from build123d import *

# Parameters (mm, degrees)
SKETCH1_R   = 6
SKETCH1_R_2 = 1.25
MAIN_DEPTH  = 8
SKETCH4_R   = 2.5


with BuildPart() as part:
    # Sketch1 → Main (new body)
    with BuildSketch(Plane.XY):
        Circle(SKETCH1_R)
        Circle(SKETCH1_R_2, mode=Mode.SUBTRACT)
    extrude(amount=MAIN_DEPTH)

    # Sketch3 → TopMain (revolve)
    with BuildSketch(Plane(origin=(0, 0, 0), x_dir=(0, 0, -1), z_dir=(1, 0, 0))):
        with BuildLine():
            Line((-8, 0), (-14, 0))
            ThreePointArc((-14, 0), (-12.242640687, -4.242640687), (-8, -6))
            Line((-8, -6), (-8, 0))
        make_face()
    revolve(axis=Axis((0, 0, 10.5), (0, 0, -1)))

    # Sketch4 → HookHole (revolve, cut)
    with BuildSketch(Plane(origin=(0, 0, 0), x_dir=(0, 0, -1), z_dir=(1, 0, 0))):
        with Locations((-7, 0)):
            Circle(SKETCH4_R)
    revolve(axis=Axis((0, 6.6, 13), (0, -1, 0)), mode=Mode.SUBTRACT)


solid = part.part
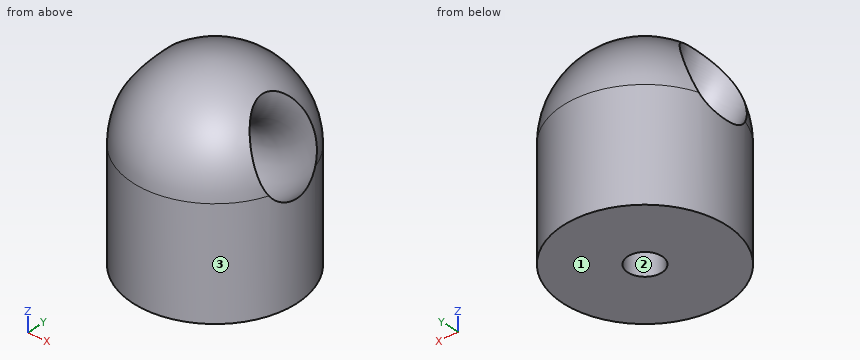
Can you work these out from the model? Positions are in its coordinate system, mm. Face numbers are marked on the shaded views. Coordinates: 2 decimals unless noted, no trailing zeros. Write each loop counter-clockwise with the first axis right and the second up, starting at its lowest first coordinate (ties: lowest second). Pieces come first, ordered by that corner, then holes. Notation, with made-up numbers: (-28.75, 25.5) -> (19.25, 25.5) arc R35 ccw to (19.25, 60.5) -> close; hole circle Ø9 at (74, 20.25). An arc over 180 degrees is marked (long way). Write item = value, one per line.
(1) Imagine slicing it at A-A (y = 0). Please give me the cut outline in (x, z) (3 decimals).
Verdict:
outline = (-6, 0) -> (-1.25, 0) -> (-1.25, 4.592) arc R8.5 cw to (-6, 6.979) -> close; (-3.498, 12.875) arc R3.5 ccw to (3.498, 12.875) arc R6 ccw to start; (1.25, 0) -> (6, 0) -> (6, 6.979) arc R8.5 cw to (1.25, 4.592) -> close
(2) For pin 1 (5 mm diameter, centred on x = -4, y = -3, fed in from +Z); pin 2 (4 mm diameter, centred on y = 2.5, z = 11, fed in from -X); pin 3 (4 mm diameter, centred on y = -2.5, z = 4.5, fed in from -X); pin 4 (6 mm diameter, centred on y = -1, z = 3, fed in from +X), each with a flat end and sliding along its axis, tell me the tip position at first contact or that it passes through.
Verdict:
pin_1 = 13.45
pin_2 = -5.41
pin_3 = -5.98
pin_4 = 6
(3) Imagine slicing it at B-B (z = 3.5). Please give me the cut outline in (x, y), and give its area (3 significant figures).
Verdict:
outline = circle Ø12 at (0, 0); hole circle Ø2.5 at (0, 0)
area = 108 mm^2
(4) Thinking about a two-plate mould opening in X: for the marked faces 1, 2 and 3, which applies, +X half, -X half, draft (parallel to the pull), parting line (faces both ways), or undercut?
Verdict:
face_1 = draft
face_2 = undercut
face_3 = parting line
(5) If I drill on probe 1 along X at (y, z) = (0, 3.2); probe 2 along Y at (x, z) = (2.75, 10.5), over which ranges is the centre line in solid material (lowest first)?
Verdict:
probe_1 = -6 to -1.25, 1.25 to 6
probe_2 = -4.71 to -1.02, 1.02 to 4.71
